Geometry: see drawing. Coordinates: mm, zero at the bounding-box minimum. A direction names the side the tool comes from. Round coordinates to 2 decimals unless told otherwise and drop trailing zeros. Write each loop counter-clockwise with the first axis right and the second up, starting at its lowest first coordinate (ties: lowest second). Pieces come first, ordered by that corner, then holes. Notation, with made-up numbers: M 11,-38.5 L 18,-38.5 A30 cw 18,-16.5 Z; hole C 3,-30.5 d4. An arc over 180 degrees is marked long. Use one line per item in the form item = value. Start each with the question number.
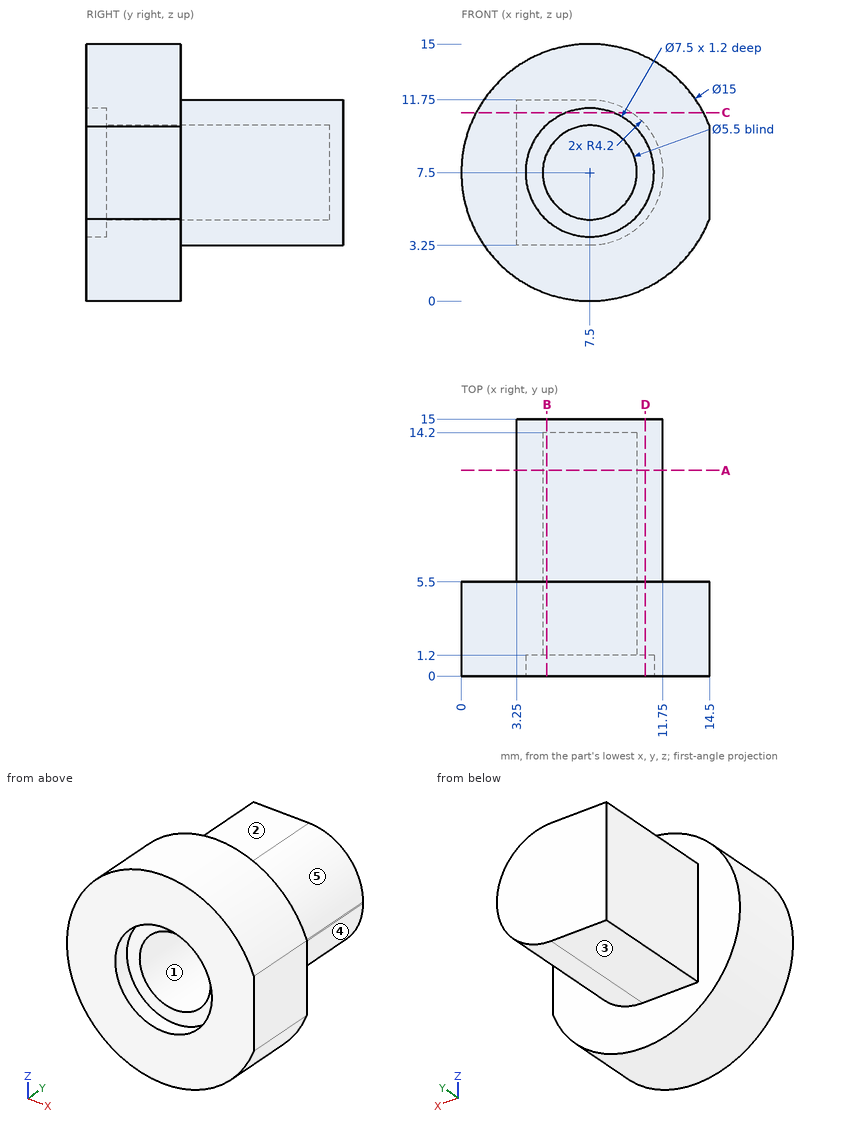
Item 1: Cut plane C-C (z = 11). Output: boundary loops of the cut face in (x, y), plus the area to 3 significant figures.
Item 2: Reachability of the marked faces 1, 2, 3, 4 and 5 from +Z, -Z, +X, -X, +Y, -Y: full face, straight path, thin tool, end or side. Return the list, or none.
Item 3: Ray query, line 1 (X direction, y = 0.65, z = 7.5); line 2 (X direction, y = 13.75, z = 7.5); line 3 (Y direction, x = 9, z = 8). Return the intervals inside material, ascending. Write a range as from..to.
Item 4: Cut plane D-D (x = 10.75). Output: boundary loops of the cut face in (y, z).
Item 5: First-contact query: pin 1 (4 mm diameter, centred on y = 10.5, z = 6.5, fed in from -X); pin 2 (1 mm diameter, centred on y = 4.5, z = 11.5, fed in from +X); pin 3 (7 mm diameter, centred on x = 7.5, z = 7.5, fed in from -Y). Flat tips, straight axial feed; report the tip coordinate or a pass-through.
Item 6: Cut plane B-B (x = 5). Output: boundary loops of the cut face in (y, z), plus the area to 3 significant figures.
Item 7: Cut plane A-A (y = 12). Output: boundary loops of the cut face in (x, z), plus the area to 3 significant figures.
Final values:
q1.outline = M 0.87,0 L 6.15,0 L 6.15,1.2 L 8.85,1.2 L 8.85,0 L 14.13,0 L 14.13,5.5 L 9.95,5.5 L 9.95,15 L 3.25,15 L 3.25,5.5 L 0.87,5.5 Z
q1.area = 133 mm^2
q2.face_1 = -Y
q2.face_2 = +Z, +X, -X, +Y
q2.face_3 = -Z, +X, -X, +Y
q2.face_4 = -Z, +X, +Y
q2.face_5 = +Z, +X, +Y
q3.line_1 = 0..3.75, 11.25..14.5
q3.line_2 = 3.25..4.75, 10.25..11.75
q3.line_3 = 14.2..15
q4.outline = M 0,0.74 L 5.5,0.74 L 5.5,4.73 L 15,4.73 L 15,10.27 L 5.5,10.27 L 5.5,14.26 L 0,14.26 L 0,9.37 L 1.2,9.37 L 1.2,5.63 L 0,5.63 Z
q5.pin_1 = 3.25
q5.pin_2 = 14.13
q5.pin_3 = 1.2
q6.outline = M 0,0.43 L 5.5,0.43 L 5.5,3.25 L 15,3.25 L 15,11.75 L 5.5,11.75 L 5.5,14.57 L 0,14.57 L 0,10.3 L 1.2,10.3 L 1.2,8.65 L 14.2,8.65 L 14.2,6.35 L 1.2,6.35 L 1.2,4.7 L 0,4.7 Z
q6.area = 122 mm^2
q7.outline = M 3.25,3.25 L 7.55,3.25 A4.2 ccw 11.75,7.45 L 11.75,7.55 A4.2 ccw 7.55,11.75 L 3.25,11.75 Z; hole C 7.5,7.5 d5.5
q7.area = 40.9 mm^2
